```python
from build123d import *

# Parameters (mm, degrees)
SKETCH1_W           = 12
SKETCH1_H           = 12
BOSS_EXTRUDE1_DEPTH = 5.5
SKETCH2_W           = 11
SKETCH2_H           = 11
CUT_EXTRUDE1_DEPTH  = 5
SKETCH3_W           = 4.8
SKETCH3_H           = 4.8
BOSS_EXTRUDE2_DEPTH = 2.2
SKETCH4_W           = 0.5
SKETCH4_H           = 3.8
BOSS_EXTRUDE3_DEPTH = 2.8
SKETCH5_W           = 0.5
SKETCH5_H           = 3.8
BOSS_EXTRUDE4_DEPTH = 2.8


with BuildPart() as part:
    # Sketch1 → Boss-Extrude1 (new body)
    with BuildSketch(Plane(origin=(0, 0, 0), x_dir=(1, 0, 0), z_dir=(0, 1, 0))):
        Rectangle(SKETCH1_W, SKETCH1_H)
    extrude(amount=-BOSS_EXTRUDE1_DEPTH)

    # Sketch2 → Cut-Extrude1 (cut)
    with BuildSketch(Plane.XZ.offset(5.5)):
        Rectangle(SKETCH2_W, SKETCH2_H)
    extrude(amount=-CUT_EXTRUDE1_DEPTH, mode=Mode.SUBTRACT)

    # Sketch3 → Boss-Extrude2 (add)
    with BuildSketch(Plane.XZ.offset(0.5)):
        Rectangle(SKETCH3_W, SKETCH3_H)
    extrude(amount=BOSS_EXTRUDE2_DEPTH)

    # Sketch4 → Boss-Extrude3 (add)
    with BuildSketch(Plane.XZ.offset(2.7)):
        with Locations((-2.15, 0)):
            Rectangle(SKETCH4_W, SKETCH4_H)
    extrude(amount=BOSS_EXTRUDE3_DEPTH)

    # Sketch5 → Boss-Extrude4 (add)
    with BuildSketch(Plane.XZ.offset(2.7)):
        with Locations((2.15, 0)):
            Rectangle(SKETCH5_W, SKETCH5_H)
    extrude(amount=BOSS_EXTRUDE4_DEPTH)


solid = part.part
```
Work out the finished part from the listing and answer in its coordinate system (mm). A direction names the side the tool comes from. Coordinates: 2 decimals unless noted, no trailing zeros. Write each loop counter-clockwise with the first axis right and the second up, starting at its lowest first coordinate (ties: lowest second). Pieces come first, ordered by that corner, then holes.
Q1. A cutting plane is placed at A-A, the plane y = -3.45. Give the vertices of the cut face in (x, z), then the cut area to 3 significant figures.
Q2. Each of these flat-tipped pins is pushed along its axis until it touches: pin 1 Ø6 at (x, z) = (3.5, 4.5) entering from -Y; pin 2 Ø1.4 at (x, z) = (0.5, 0) entering from -Y. Where does it stop, or does it pass through?
Q3. A cutting plane is placed at D-D, the plane x = 3. Give the vertices of the cut face in (y, z).
Q4. Which of the six approach directions +Z, -Z, +X, -X, +Y, -Y give full straight-line access (tool end or side, diameter ignored) to faces 1 (the face through (-0.5, -5.5, 5.7)), 2 (the face through (0, -2, -2.4))?
Q5. Determine the mould class of faces 3 (the face through (2.4, -3, 0)), 4 (the face through (0, -3, 6)), 5 (the face through (-6, -3, 0)) for opening direction Z: released by +Z, released by -Z, zero draft, split by the parting line, or undercut.
Q6. A cutting plane is placed at C-C, the plane z = -0.5. Give the vertices of the cut face in (x, y), then the cut area to 3 significant figures.
Q7. A cutting plane is placed at B-B, the plane y = -1.55. Give the vertices of the cut face in (x, z), then the cut area to 3 significant figures.
Q8. Find the intervals of material crossed by line 1 (Z direction, x = 0.75, y = -2.6); line 2 (X direction, y = -3.85, z = -1), in increasing order.
Findings below:
1. outline: (-6, -6) - (6, -6) - (6, 6) - (-6, 6) - close; (-2.4, -1.9) - (-1.9, -1.9) - (-1.9, 1.9) - (-2.4, 1.9) - close; (1.9, -1.9) - (2.4, -1.9) - (2.4, 1.9) - (1.9, 1.9) - close; hole (-5.5, -5.5) - (5.5, -5.5) - (5.5, 5.5) - (-5.5, 5.5) - close
1. area: 26.8 mm2
2. pin 1: stops at y = -5.5
2. pin 2: stops at y = -2.7
3. outline: (-5.5, -6) - (0, -6) - (0, 6) - (-5.5, 6) - (-5.5, 5.5) - (-0.5, 5.5) - (-0.5, -5.5) - (-5.5, -5.5) - close
4. face 1: +Z, -Z, +X, -X, -Y
4. face 2: -Y
5. face 3: undercut
5. face 4: released by +Z
5. face 5: zero draft
6. outline: (-6, -5.5) - (-5.5, -5.5) - (-5.5, -0.5) - (-2.4, -0.5) - (-2.4, -5.5) - (-1.9, -5.5) - (-1.9, -2.7) - (1.9, -2.7) - (1.9, -5.5) - (2.4, -5.5) - (2.4, -0.5) - (5.5, -0.5) - (5.5, -5.5) - (6, -5.5) - (6, 0) - (-6, 0) - close
6. area: 24.4 mm2
7. outline: (-6, -6) - (6, -6) - (6, 6) - (-6, 6) - close; (-2.4, -2.4) - (2.4, -2.4) - (2.4, 2.4) - (-2.4, 2.4) - close; hole (-5.5, -5.5) - (5.5, -5.5) - (5.5, 5.5) - (-5.5, 5.5) - close
7. area: 46.0 mm2
8. line 1: z = -6 to -5.5, -2.4 to 2.4, 5.5 to 6
8. line 2: x = -6 to -5.5, -2.4 to -1.9, 1.9 to 2.4, 5.5 to 6
